from build123d import *

# Parameters (mm, degrees)
SKETCH_1_W          = 70
SKETCH_1_H          = 70
EXTRUDE_1_DEPTH     = 4
SKETCH_2_R          = 1.575
CUT_EXTRUDE_1_DEPTH = 100.075728612
FILLET_1_R          = 15


with BuildPart() as part:
    # 草图1 → 凸台-拉伸1 (new body)
    with BuildSketch(Plane.XY):
        with Locations((35, -35)):
            Rectangle(SKETCH_1_W, SKETCH_1_H)
    extrude(amount=EXTRUDE_1_DEPTH)

    # 草图2 → 切除-拉伸1 (cut, through all)
    with BuildSketch(Plane.XY.offset(4)):
        with Locations((27.5, -10)):
            Circle(SKETCH_2_R)
        with Locations(Location((42.5, -10, 0), (0, 0, 180))):
            Circle(SKETCH_2_R)
        with Locations((42.5, -20)):
            Circle(SKETCH_2_R)
        with Locations(Location((27.5, -20, 0), (0, 0, 180))):
            Circle(SKETCH_2_R)
        with Locations((27.5, -50)):
            Circle(SKETCH_2_R)
        with Locations(Location((42.5, -50, 0), (0, 0, 180))):
            Circle(SKETCH_2_R)
        with Locations((42.5, -60)):
            Circle(SKETCH_2_R)
        with Locations(Location((27.5, -60, 0), (0, 0, 180))):
            Circle(SKETCH_2_R)
        with Locations((13.433243174, -13.433243174)):
            Circle(SKETCH_2_R)
        with Locations((56.566756826, -13.433243174)):
            Circle(SKETCH_2_R)
        with Locations((56.566756826, -56.566756826)):
            Circle(SKETCH_2_R)
        with Locations((13.433243174, -56.566756826)):
            Circle(SKETCH_2_R)
        Polygon((21, -29), (15.803847577, -32), (15.803847577, -38), (21, -41), (26.196152423, -38), (26.196152423, -32), align=None)
        Polygon((35, -41), (40.196152423, -38), (40.196152423, -32), (35, -29), (29.803847577, -32), (29.803847577, -38), align=None)
        Polygon((43.803847577, -38), (43.803847577, -32), (49, -29), (54.196152423, -32), (54.196152423, -38), (49, -41), align=None)
    extrude(amount=-CUT_EXTRUDE_1_DEPTH, mode=Mode.SUBTRACT)

    # 圆角1
    fillet_1_edges = [part.edges().sort_by_distance(p)[0] for p in [
        (0, 0, 2),
        (70, 0, 2),
        (70, -70, 2),
        (0, -70, 2),
    ]]
    fillet(fillet_1_edges, radius=FILLET_1_R)


solid = part.part
CAD build for the part. Positions are in the model's coordinates, mm. A direction names the side the tool comes from. Round coordinates to 2 decimals unless told otherwise and drop trailing zeros. Write each loop counter-clockwise with the first axis right and the second up, starting at its lowest first coordinate (ties: lowest second). Pieces come first, ordered by that corner, then holes. Notation, with made-up numbers: (-35, -33.5) -> (-18, -33.5) arc R19 ccw to (-18, -2.5) -> close; hole circle Ø5 at (10.5, -24.75). An arc over 180 degrees is marked (long way). Answer as a JSON object with one key per item and string values.
(1) Probe probe 1 along X at (y, z) = (-34, 0.6); probe 2 along Y at (x, z) = (42.5, 1) (3 decimals); probe 3 along X at (y, z) = (-39, 3.45). List the from-to ranges inside material, lowest first. Write a range as [from, to].
Reported:
{"probe 1": "x = [0, 15.8], [26.2, 29.8], [40.2, 43.8], [54.2, 70]", "probe 2": "y = [-70, -61.575], [-58.425, -51.575], [-48.425, -21.575], [-18.425, -11.575], [-8.425, 0]", "probe 3": "x = [0, 17.54], [24.46, 31.54], [38.46, 45.54], [52.46, 70]"}
(2) Which spindle directions (+Z, -Z, +X, -X, +Y, -Y) get a long thin tool onto all of the face, cutting with end or side? Do faces 4 (the face through (65.49, -65.72, 2.03)), 5 (the face through (40.196, -35, 2)). Say none if no direction does.
Reported:
{"face 4": "+Z, -Z, +X, -Y", "face 5": "+Z, -Z"}
(3) Two-plate mould, pull along X, no slides. Class faces 1 (the face through (18.4, -30.5, 2)), 2 (the face through (35, -70, 2)), 3 (the face through (70, -35, 2)): +X half, -X half, draft (parallel to the pull), parting line (faces both ways), or undercut.
Reported:
{"face 1": "undercut", "face 2": "draft", "face 3": "+X half"}
(4) Band-saw the part on A-A, the plane y = -20. List the corners of the cut face in (x, z) (3 decimals), then the cut area to 3 significant figures.
Reported:
{"outline": "(0, 0) -> (25.925, 0) -> (25.925, 4) -> (0, 4) -> close; (29.075, 0) -> (40.925, 0) -> (40.925, 4) -> (29.075, 4) -> close; (44.075, 0) -> (70, 0) -> (70, 4) -> (44.075, 4) -> close", "area": "255 mm^2"}
(5) Band-saw the part on D-D, the plane y = -34. List the corners of the cut face in (x, z).
Reported:
{"outline": "(0, 0) -> (15.8, 0) -> (15.8, 4) -> (0, 4) -> close; (26.2, 0) -> (29.8, 0) -> (29.8, 4) -> (26.2, 4) -> close; (40.2, 0) -> (43.8, 0) -> (43.8, 4) -> (40.2, 4) -> close; (54.2, 0) -> (70, 0) -> (70, 4) -> (54.2, 4) -> close"}
(6) Band-saw the part on C-C, the plane x = 38. List the corners of the cut face in (y, z), then the cut area to 3 significant figures.
Reported:
{"outline": "(-70, 0) -> (-39.27, 0) -> (-39.27, 4) -> (-70, 4) -> close; (-30.73, 0) -> (0, 0) -> (0, 4) -> (-30.73, 4) -> close", "area": "246 mm^2"}
(7) Band-saw the part on B-B, the plane x = 27.5. List the corners of the cut face in (y, z) (3 decimals), then the cut area to 3 significant figures.
Reported:
{"outline": "(-70, 0) -> (-61.575, 0) -> (-61.575, 4) -> (-70, 4) -> close; (-58.425, 0) -> (-51.575, 0) -> (-51.575, 4) -> (-58.425, 4) -> close; (-48.425, 0) -> (-21.575, 0) -> (-21.575, 4) -> (-48.425, 4) -> close; (-18.425, 0) -> (-11.575, 0) -> (-11.575, 4) -> (-18.425, 4) -> close; (-8.425, 0) -> (0, 0) -> (0, 4) -> (-8.425, 4) -> close", "area": "230 mm^2"}
